```python
from build123d import *

# Parameters (mm, degrees)
ENL_V_MAT_EXTRU_1_DEPTH      = 7.5
ENL_V_MAT_EXTRU_1_DEPTH_BACK = 7.5
BOSS_EXTRU_1_REACH           = 27.5
ECHELLE1_SCALE               = 1.8


with BuildPart() as part:
    # Esquisse1 → R_volution1 (revolve)
    with BuildSketch(Plane.XY):
        with BuildLine():
            Line((0, 0), (0, 100))
            Line((0, 100), (-18, 100))
            Line((-18, 100), (-7.593007693, 6.792401612))
            ThreePointArc((-7.593007693, 6.792401612), (-5.093880777, 1.945904787), (0, 0))
        make_face()
    revolve(axis=Axis((0, 0, 0), (0, 1, 0)))

    # Esquisse2 → Enl_v. mat.-Extru.1 (cut, two sides)
    with BuildSketch(Plane.XY) as enl_v_mat_extru_1_sk:
        with BuildLine():
            Line((-13.5, 100), (13.5, 100))
            add(Edge.make_bspline(
                [(-13.5, 100), (-13.291113541, 83.520875666), (13.291113541, 83.520875666), (13.5, 100)],
                knots=[0, 0, 0, 0, 1, 1, 1, 1], degree=3))
        make_face()
    extrude(amount=ENL_V_MAT_EXTRU_1_DEPTH, mode=Mode.SUBTRACT)
    extrude(enl_v_mat_extru_1_sk.sketch, amount=-ENL_V_MAT_EXTRU_1_DEPTH_BACK, mode=Mode.SUBTRACT)

    # Esquisse3 → Boss.-Extru.1 (add, up to next)
    with BuildSketch(Plane.XY.offset(-7.5), mode=Mode.PRIVATE) as boss_extru_1_sk1:
        with BuildLine():
            Line((-5, 100), (5, 100))
            add(Edge.make_bspline(
                [(-5, 100), (0, 91.498247822), (5, 100)],
                knots=[0, 0, 0, 1, 1, 1], degree=2))
        make_face()
    boss_extru_1_tool1 = extrude(boss_extru_1_sk1.sketch, amount=BOSS_EXTRU_1_REACH, mode=Mode.PRIVATE) - part.part
    add(boss_extru_1_tool1.solids().sort_by_distance((0, 98.29965, -7.5))[0])


with BuildPart() as part_1:
    # Echelle1: scaled about (-4e-09, 62.219241992, 3e-09)
    add(part.part.scale(ECHELLE1_SCALE).moved(Location((3e-09, -49.775393594, -2e-09))))


solid = part_1.part
```
Geometry check sheet. Reference: the model listing, model coordinates, mm. Coordinates: 2 decimals unless noted, no trailing zeros. Loops run counter-clockwise (first coordinate to the right, second up) from the corner with the lowest first, then second, coordinate; pieces in that order, holes last.
Item 1: Thickness scan on line 1 (X direction, y = 59, z = -2.5); line 2 (Z direction, x = 1, y = 119); line 3 (Z direction, x = -14.5, y = 117). Record the ranges inside material, lowest first.
Item 2: Sectioned sample at A-A, the plane y = 69.5. Record the boundary of the cut face in (x, z), then the cut area to 3 significant figures.
Item 3: Sectioned sample at B-B, the plane y = 20. Record the boundary of the cut face in (x, z), then the cut area to 3 significant figures.
Item 4: Go/stop test with flat-tipped pins: pin 1 Ø3 at (y, z) = (52, -7) entering from -X; pin 2 Ø12 at (y, z) = (64, 18.5) entering from -X; pin 3 Ø12 at (y, z) = (22.5, -13) entering from +X. Record where each tip stops, or that it passes through.
Item 5: Release check for a two-part mould opening along Z. For faces 1 (the face through (0, 130.225, 0)), 2 (the face through (16.88, 45.16, 15.48)), 3 (the face through (0, 119, 13.5)) record: released by +Z, released by -Z, zero draft, split by the parting line, or undercut.
Check result:
1. line 1: x = -24.32 to 24.32
1. line 2: z = -31.13 to -13.5, 13.5 to 31.13
1. line 3: z = -27.31 to -13.5, 13.5 to 27.31
2. outline: circle Ø51.24 at (0, 0)
2. area: 2,060 mm2
3. outline: circle Ø40.19 at (0, 0)
3. area: 1,270 mm2
4. pin 1: stops at x = -23.06
4. pin 2: stops at x = -21.74
4. pin 3: stops at x = 19.24
5. face 1: zero draft
5. face 2: split by the parting line
5. face 3: undercut
